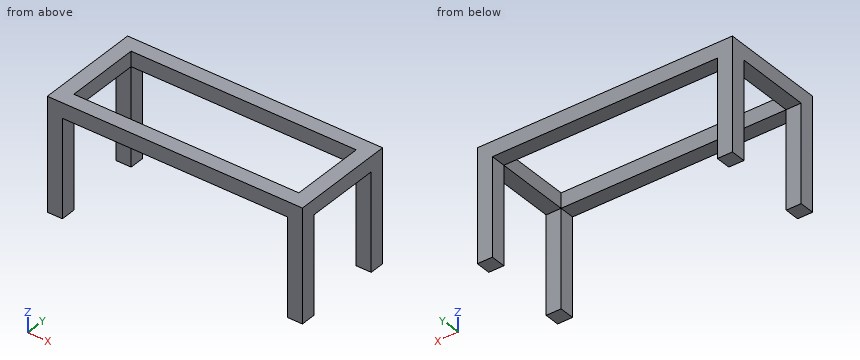
from build123d import *

# Parameters (mm, degrees)
F0_W     = 215.9
F0_H     = 88.9
F1_DEPTH = 95.25
F2_W     = 190.5
F2_H     = 63.5
F3_DEPTH = 95.251
F4_W     = 190.5
F4_H     = 82.55
F5_DEPTH = 88.901
F6_W     = 63.5
F6_H     = 82.55
F7_DEPTH = 215.901


with BuildPart() as f1:
    # F0 (on Top) → F1 (new body)
    with BuildSketch(Plane.XY):
        with Locations((-116.891209875, 41.7768546164)):
            Rectangle(F0_W, F0_H)
    extrude(amount=F1_DEPTH)

    # F2 (on face) → F3 (cut, through all)
    with BuildSketch(Plane.XY.offset(95.25)):
        with Locations((-116.891209875, 41.7768546164)):
            Rectangle(F2_W, F2_H)
    extrude(amount=-F3_DEPTH, mode=Mode.SUBTRACT)

    # F4 (on face) → F5 (cut, through all)
    with BuildSketch(Plane.XZ.offset(2.6731453836)):
        with Locations((-116.891209875, 41.275)):
            Rectangle(F4_W, F4_H)
    extrude(amount=-F5_DEPTH, mode=Mode.SUBTRACT)

    # F6 (on face) → F7 (cut, through all)
    with BuildSketch(Plane.YZ.offset(-8.941209875)):
        with Locations((41.7768546164, 41.275)):
            Rectangle(F6_W, F6_H)
    extrude(amount=-F7_DEPTH, mode=Mode.SUBTRACT)


solid = f1.part
The listing builds one solid part. Answer for the finished solid, in the listing's coordinates (mm). Give positions to 0.01 mm unless a question says otherwise; leave off trailing zeros. Loops run counter-clockwise (first coordinate to the right, second up) from the corner with the lowest first, then second, coordinate; pieces in that order, holes last. Notation, with made-up numbers: (72.25, 68.5) - (82.25, 68.5) arc R33 ccw to (82.25, 105.5) - close; hole circle Ø10 at (23.5, -27). An arc over 180 degrees is marked (long way). Write each question's results on one line, items separated by ' | '.
1. Find section C-C, the plane z = 73.5. Write down the section's boundary in (x, y), then the cut area to 3 significant figures.
Resolved:
outline: (-224.84, -2.67) - (-212.14, -2.67) - (-212.14, 10.03) - (-224.84, 10.03) - close; (-224.84, 73.53) - (-212.14, 73.53) - (-212.14, 86.23) - (-224.84, 86.23) - close; (-21.64, -2.67) - (-8.94, -2.67) - (-8.94, 10.03) - (-21.64, 10.03) - close; (-21.64, 73.53) - (-8.94, 73.53) - (-8.94, 86.23) - (-21.64, 86.23) - close | area: 645 mm^2
2. Find section B-B, the plane y = 47. Write down the section's boundary in (x, z).
Resolved:
outline: (-224.84, 82.55) - (-212.14, 82.55) - (-212.14, 95.25) - (-224.84, 95.25) - close; (-21.64, 82.55) - (-8.94, 82.55) - (-8.94, 95.25) - (-21.64, 95.25) - close
3. Find section D-D, the plane y = 3.5. Write down the section's boundary in (x, z).
Resolved:
outline: (-224.84, 0) - (-212.14, 0) - (-212.14, 82.55) - (-21.64, 82.55) - (-21.64, 0) - (-8.94, 0) - (-8.94, 95.25) - (-224.84, 95.25) - close
4. A flat-ended cylindrical pin translates along its axis: P1, Ø10, axis at x = -82.5, y = 77.5, coming from the -Z side. Find the tip coordinate at first contact, or state that the pin passes through.
Resolved:
P1: stops at z = 82.55
5. Consider probe 1 along Y at (x, z) = (-214.5, 32); probe 2 along X at (y, z) = (80, 60.5); probe 3 along Z at (x, y) = (-189, 76). Determine where each line is inside the solid, lowest interval first. Write a range as from..to.
Resolved:
probe 1: y = -2.67..10.03, 73.53..86.23 | probe 2: x = -224.84..-212.14, -21.64..-8.94 | probe 3: z = 82.55..95.25
6. Find section A-A, the plane x = -92.5. Write down the section's boundary in (y, z), then the cut area to 3 significant figures.
Resolved:
outline: (-2.67, 82.55) - (10.03, 82.55) - (10.03, 95.25) - (-2.67, 95.25) - close; (73.53, 82.55) - (86.23, 82.55) - (86.23, 95.25) - (73.53, 95.25) - close | area: 323 mm^2
